```python
from build123d import *

# Parameters (mm, degrees)
SKETCH1_W           = 60
SKETCH1_H           = 100
BOSS_EXTRUDE1_DEPTH = 3
BOSS_EXTRUDE2_DEPTH = 60
BOSS_EXTRUDE3_START = -5
SKETCH3_W           = 5
SKETCH3_H           = 2.614864802
BOSS_EXTRUDE3_DEPTH = 5


with BuildPart() as part:
    # Sketch1 → Boss-Extrude1 (new body)
    with BuildSketch(Plane(origin=(0, 0, 0), x_dir=(1, 0, 0), z_dir=(0, 1, 0))):
        Rectangle(SKETCH1_W, SKETCH1_H)
    extrude(amount=BOSS_EXTRUDE1_DEPTH)

    # Sketch2 → Boss-Extrude2 (add)
    with BuildSketch(Plane(origin=(0, 3, 0), x_dir=(1, 0, 0), z_dir=(0, 1, 0))):
        Polygon((-9.5, 2.5), (-7, 2.5), (-7, 7.5), (-12, 7.5), (-12, 2.5), align=None)
        Polygon((-9.5, -2.5), (-7, -2.5), (-7, -7.5), (-12, -7.5), (-12, -2.5), align=None)
    extrude(amount=BOSS_EXTRUDE2_DEPTH)

    # Sketch3 → Boss-Extrude3 (add)
    with BuildSketch(Plane(origin=(-7, 0, 0), x_dir=(0, 0, -1), z_dir=(1, 0, 0)).offset(BOSS_EXTRUDE3_START)):
        with Locations((0, 21.692567599)):
            Rectangle(SKETCH3_W, SKETCH3_H)
    extrude(amount=BOSS_EXTRUDE3_DEPTH)


solid = part.part
```
The listing builds one solid part. Answer for the finished solid, in the listing's coordinates (mm). A direction names the side the tool comes from. Round coordinates to 2 decimals unless told otherwise and drop trailing zeros. Loops run counter-clockwise (first coordinate to the right, second up) from the corner with the lowest first, then second, coordinate; pieces in that order, holes last. Notation, with made-up numbers: (15.5, 64.25) - (55.5, 64.25) arc R25 ccw to (55.5, 103.25) - close; hole circle Ø5 at (77, -7.75). An arc over 180 degrees is marked (long way). Return JSON: item names as keys, results as strings. Group by question number.
1. The mould has two halves that part along Z. Classify faces 4 (the flat face through (-10, 20.385, 0)), 5 (the flat face through (0, 1, 50)), 6 (the flat face through (0, 0, -1)): pulls with the +Z half, pulls with the -Z half, needs draft (parallel to the pull), parting line crosses it, or undercut.
2. The part is cut by section D-D on z = -25. Determine the outline of the cut face in (x, y), then the cut area to 3 significant figures.
3. Consider probe 1 along Z at (x, y) = (-9.5, 14); probe 2 along Y at (x, z) = (0.5, 39.5). Determine where each line is inside the solid, lowest interval first.
4. The part is cut by section B-B on z = -4. Determine the outline of the cut face in (x, y), then the cut area to 3 significant figures.
5. The part is cut by section A-A on y = 45. Determine the outline of the cut face in (x, z), then the cut area to 3 significant figures.
6. The part is cut by section C-C on x = 15.5. Determine the outline of the cut face in (y, z).
7. Which of the six approach directions +Z, -Z, +X, -X, +Y, -Y give full straight-line access (tool end or side, diameter ignored) to faces 1 (the flat face through (-9, 12, 2.5)), 2 (the flat face through (-10, 23, 0)), 3 (the flat face through (-9, 33, 7.5))?
8. Each of these flat-tipped pins is pushed along its axis until it touches: P1, Ø1.5, axis at x = -10, y = 48, coming from the -Z side; P2, Ø10, axis at x = -17, z = 16, coming from the +Y side; P3, Ø4, axis at x = -8.5, y = 34.5, coming from the +Z side; P4, Ø3, axis at x = 17, z = 4.5, coming from the -Y side. Where does it stop, or does it pass through?
Resolved:
{
 "1": {"face 4": "undercut", "face 5": "pulls with the +Z half", "face 6": "needs draft"},
 "2": {"outline": "(-30, 0) - (30, 0) - (30, 3) - (-30, 3) - close", "area": "180 mm²"},
 "3": {"probe 1": "z = -7.5 to -2.5, 2.5 to 7.5", "probe 2": "y = 0 to 3"},
 "4": {"outline": "(-30, 0) - (30, 0) - (30, 3) - (-7, 3) - (-7, 63) - (-12, 63) - (-12, 3) - (-30, 3) - close", "area": "480 mm²"},
 "5": {"outline": "(-12, -7.5) - (-7, -7.5) - (-7, -2.5) - (-12, -2.5) - close; (-12, 2.5) - (-7, 2.5) - (-7, 7.5) - (-12, 7.5) - close", "area": "50.0 mm²"},
 "6": {"outline": "(0, -50) - (3, -50) - (3, 50) - (0, 50) - close"},
 "7": {"face 1": "+X, -X", "face 2": "+X, -X, +Y", "face 3": "+Z, +X, -X, +Y"},
 "8": {"P1": "stops at z = -7.5", "P2": "stops at y = 3", "P3": "stops at z = 7.5", "P4": "stops at y = 0"}
}
